from build123d import *
from build123d.topology import SkipClean

# Parameters (mm, degrees)
BOSS_EXTRUDE1_DEPTH                        = 2
BOSS_EXTRUDE2_DEPTH                        = 12.7
BOSS_EXTRUDE2_DEPTH_BACK                   = 2
SKETCH2_W                                  = 38.1
SKETCH2_H                                  = 44.1
SKETCH2_W_2                                = 34.1
SKETCH2_H_2                                = 40.1
SKETCH4_W                                  = 17.8
SKETCH4_H                                  = 2
SKETCH4_W_2                                = 23
CUT_EXTRUDE1_DEPTH                         = 8
SKETCH5_W                                  = 5
SKETCH5_H                                  = 6.5
BOSS_EXTRUDE3_DEPTH                        = 11.05
SKETCH3_R                                  = 1.05
CUT_EXTRUDE2_DEPTH                         = 33.637325258
MIRROR1_AT_THE_SECOND_PLANE_COPY_1_SKETC_R = 1.05
MIRROR1_AT_THE_SECOND_PLANE_COPY_1_DEPTH   = 33.637325258


with BuildPart() as part:
    # Sketch1 → Boss-Extrude1 (new body)
    with BuildSketch(Plane(origin=(0, 0, 0), x_dir=(1, 0, 0), z_dir=(0, 1, 0))):
        Polygon((-17.05, 20.05), (-17.05, -20.05), (17.05, -20.05), align=None)
        Polygon((17.05, 20.05), (17.05, -20.05), (-17.05, 20.05), align=None)
    extrude(amount=BOSS_EXTRUDE1_DEPTH)

    # Sketch2 → Boss-Extrude2 (add, two sides: drawn at the far end of the back side and taken through both)
    with BuildSketch(Plane(origin=(0, 2, 0), x_dir=(1, 0, 0), z_dir=(0, 1, 0)).offset(-BOSS_EXTRUDE2_DEPTH_BACK)):
        Rectangle(SKETCH2_W, SKETCH2_H)
        Rectangle(SKETCH2_W_2, SKETCH2_H_2, mode=Mode.SUBTRACT)
    extrude(amount=BOSS_EXTRUDE2_DEPTH + BOSS_EXTRUDE2_DEPTH_BACK)

    # Sketch4 → Cut-Extrude1 (cut)
    with BuildSketch(Plane(origin=(0, 14.7, 0), x_dir=(1, 0, 0), z_dir=(0, 1, 0))):
        with Locations((0, 21.05)):
            Rectangle(SKETCH4_W, SKETCH4_H)
        with Locations((0, -21.05)):
            Rectangle(SKETCH4_W_2, SKETCH4_H)
    extrude(amount=-CUT_EXTRUDE1_DEPTH, mode=Mode.SUBTRACT)

    # Sketch5 → Boss-Extrude3 (add)
    with BuildSketch(Plane(origin=(0, 2, 0), x_dir=(1, 0, 0), z_dir=(0, 1, 0))):
        with BuildLine():
            ThreePointArc((-13.95, -15.5), (-15, -16.55), (-16.05, -15.5))
            Line((-16.05, -15.5), (-17.05, -15.5))
            Line((-17.05, -15.5), (-17.05, -18))
            Line((-17.05, -18), (-12.95, -18))
            Line((-12.95, -18), (-12.95, -15.5))
            Line((-12.95, -15.5), (-13.95, -15.5))
        make_face()
        with Locations((-14.55, 16.8)):
            Rectangle(SKETCH5_W, SKETCH5_H)
        with Locations((14.55, 16.8)):
            Rectangle(SKETCH5_W, SKETCH5_H)
        with BuildLine():
            Line((13.95, -15.5), (12.95, -15.5))
            Line((12.95, -15.5), (12.95, -18))
            Line((12.95, -18), (17.05, -18))
            Line((17.05, -18), (17.05, -15.5))
            Line((17.05, -15.5), (16.05, -15.5))
            ThreePointArc((16.05, -15.5), (15, -16.55), (13.95, -15.5))
        make_face()
    extrude(amount=BOSS_EXTRUDE3_DEPTH)

    # Sketch3 → Cut-Extrude2 (cut, through all)
    with BuildSketch(Plane.XZ):
        with Locations(Location((-15, 15.5, 0), (0, 0, 270))):
            Circle(SKETCH3_R)
    cut_extrude2 = extrude(amount=-CUT_EXTRUDE2_DEPTH, mode=Mode.SUBTRACT)

    # Mirror1: Cut-Extrude2 across plane
    add(cut_extrude2.mirror(Plane.XY), mode=Mode.SUBTRACT)

    # Mirror1 at the second plane: Cut-Extrude2 across plane
    with SkipClean():  # the faces are left unmerged after this step: merging them gives an invalid solid
        add(cut_extrude2.mirror(Plane(origin=(0, 0, 0), x_dir=(0, 0, 1), z_dir=(1, 0, 0))), mode=Mode.SUBTRACT)

    # Mirror1 at the second plane copy 1 sketc → Mirror1 at the second plane copy 1 (cut, through all)
    with SkipClean():  # the faces are left unmerged after this step: merging them gives an invalid solid
        with BuildSketch(Plane(origin=(0, 0, 0), x_dir=(-1, 0, 0), z_dir=(0, -1, 0))):
            with Locations(Location((-15, 15.5, 0), (0, 0, 270))):
                Circle(MIRROR1_AT_THE_SECOND_PLANE_COPY_1_SKETC_R)
        extrude(amount=-MIRROR1_AT_THE_SECOND_PLANE_COPY_1_DEPTH, mode=Mode.SUBTRACT)


solid = part.part
CAD build for the part. Positions are in the model's coordinates, mm. A direction names the side the tool comes from. Coordinates: 2 decimals unless noted, no trailing zeros. Order: outer loops, then holes, each group sorted by start corner. A loop starts at its lowest first (then second) coordinate and runs counter-clockwise, first axis right, second up.
Item 1: Band-saw the part on D-D on y = 3.5. List the corners of the cut face in (x, z), plus the area to 3 significant figures.
Check sheet entries:
outline: (-19.05, -22.05) - (19.05, -22.05) - (19.05, 22.05) - (-19.05, 22.05) - close; hole (-17.05, -13.55) - (-12.05, -13.55) - (-12.05, -20.05) - (12.05, -20.05) - (12.05, -13.55) - (17.05, -13.55) - (17.05, 15.5) - (16.05, 15.5) arc R1.05 ccw to (13.95, 15.5) - (12.95, 15.5) - (12.95, 18) - (17.05, 18) - (17.05, 20.05) - (-17.05, 20.05) - (-17.05, 18) - (-12.95, 18) - (-12.95, 15.5) - (-13.95, 15.5) arc R1.05 ccw to (-16.05, 15.5) - (-17.05, 15.5) - close; hole circle Ø2.1 at (-15, -15.5); hole circle Ø2.1 at (15, -15.5)
area: 388 mm2
Item 2: Drill centre lines: L1, parallel to Z at x = -15, y = 6.75; L2, parallel to Z at x = 15, y = 0.8; L3, parallel to Z at x = 13, y = 3.25. Where is each one in solid material? Low to high.
Check sheet entries:
L1: z = -22.05 to -16.55, -14.45 to -13.55, 16.55 to 18, 20.05 to 22.05
L2: z = -22.05 to -16.55, -14.45 to 14.45, 16.55 to 22.05
L3: z = -22.05 to -13.55, 15.5 to 18, 20.05 to 22.05
Item 3: Pin check, flat tips, straight feed: pin 1 Ø0.6 at (x, z) = (0, -21) entering from +Y; pin 2 Ø5.5 at (x, z) = (13.5, -15.5) entering from +Y. Stop position of each tip, or through.
Check sheet entries:
pin 1: stops at y = 6.7
pin 2: stops at y = 13.05
Item 4: 3-axis set-ups, long thin cutter, end or side, ignore diameter. For faces 1 (the face through (8.9, 11, -21)), 2 (the face through (-15, 7, 18)), 3 (the face through (0, 6, -22.05)), 4 (the face through (15.64, 6.43, -16.33)), 5 (the face through (11.5, 11, 21)): which of +Z, -Z, +X, -X, +Y, -Y reach the whole face in a straight line?
Check sheet entries:
face 1: +Z, -Z, +Y
face 2: +Y
face 3: -Z, +X, -X, +Y, -Y
face 4: +Y, -Y
face 5: +Z, +Y
Item 5: Band-saw the part on A-A on z = -15.5. List the corners of the cut face in (x, y), plus the area to 3 significant figures.
Check sheet entries:
outline: (-19.05, 0) - (-16.05, 0) - (-16.05, 13.05) - (-17.05, 13.05) - (-17.05, 14.7) - (-19.05, 14.7) - close; (-13.95, 0) - (13.95, 0) - (13.95, 13.05) - (12.05, 13.05) - (12.05, 2) - (-12.05, 2) - (-12.05, 13.05) - (-13.95, 13.05) - close; (16.05, 0) - (19.05, 0) - (19.05, 14.7) - (17.05, 14.7) - (17.05, 13.05) - (16.05, 13.05) - close
area: 183 mm2
Item 6: Band-saw the part on C-C on x = 15. List the corners of the cut face in (y, z).
Check sheet entries:
outline: (0, -22.05) - (14.7, -22.05) - (14.7, -20.05) - (13.05, -20.05) - (13.05, -16.55) - (0, -16.55) - close; (0, -14.45) - (13.05, -14.45) - (13.05, -13.55) - (2, -13.55) - (2, 14.45) - (0, 14.45) - close; (0, 16.55) - (13.05, 16.55) - (13.05, 18) - (2, 18) - (2, 20.05) - (14.7, 20.05) - (14.7, 22.05) - (0, 22.05) - close
Item 7: Band-saw the part on B-B on y = 8. Give the number of separate pieces and of enclosed holes in the cut face, plus the area to 3 significant figures.
Check sheet entries:
separate pieces: 2
enclosed holes: 2
area: 306 mm2
